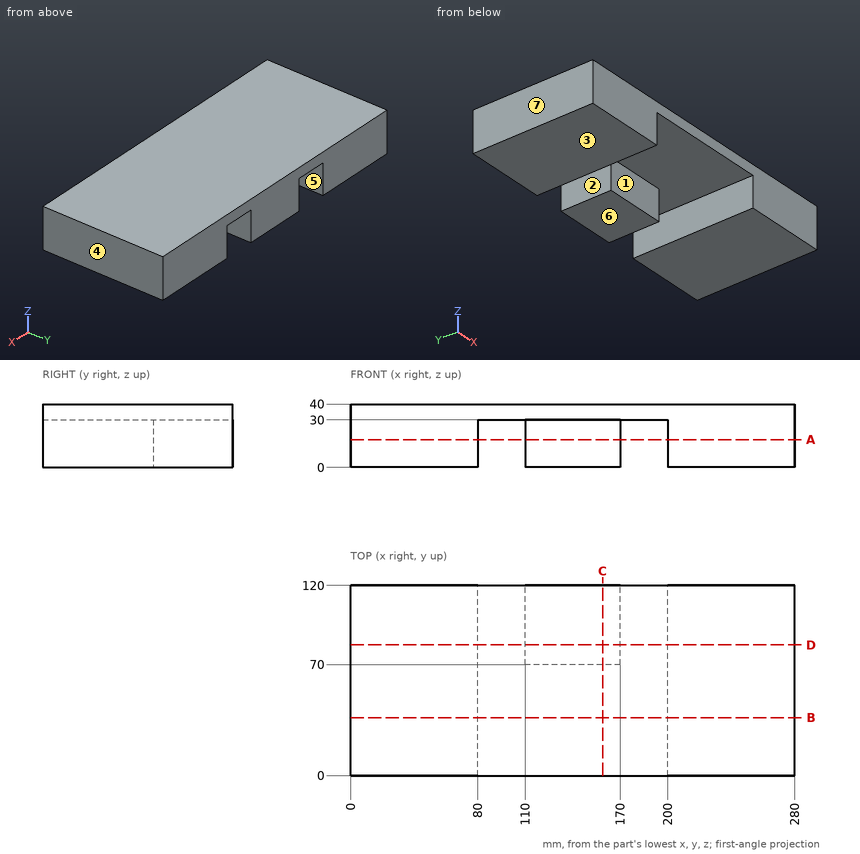
Geometry check sheet. Reference: drawing and pictorial views, mm from the part's lowest x, y, z. A direction names the side the tool comes from. Coordinates: 2 decimals unless noted, no trailing zeros. Loops run counter-clockwise (first coordinate to the right, second up) from the corner with the lowest first, then second, coordinate; pieces in that order, holes last. Notation, with made-up numbers: M 17.5,-12 L 33.5,-12 A14 cw 33.5,-8 Z; hole C 86,1.5 d10. An arc over 180 degrees is marked long. One line per item, written item: value.
1. Section check D-D on y = 82.5. Record the cut outline in (x, z).
Answers follow:
outline: M 0,0 L 80,0 L 80,30 L 110,30 L 110,0 L 170,0 L 170,30 L 200,30 L 200,0 L 280,0 L 280,40 L 0,40 Z
2. Section check A-A on z = 17.5. Record the cut outline in (x, y).
Answers follow:
outline: M 0,0 L 80,0 L 80,120 L 0,120 Z; M 110,70 L 170,70 L 170,120 L 110,120 Z; M 200,0 L 280,0 L 280,120 L 200,120 Z
3. Mould release check, pull along X, two halves, no side actions. Record for the marked faces 4, 5, 6 and 7: pulls with the +X half, pulls with the -X half, needs draft (parallel to the pull), parting line crosses it, or undercut.
Answers follow:
face 4: pulls with the +X half
face 5: undercut
face 6: needs draft
face 7: pulls with the -X half
4. Section check B-B on y = 36.5. Record the cut outline in (x, z).
Answers follow:
outline: M 0,0 L 80,0 L 80,30 L 200,30 L 200,0 L 280,0 L 280,40 L 0,40 Z
5. Gauge pin test, flat end, axial feed: P1, Ø24, axis at x = 130.5, z = 16.5, coming from the -Y side. Record the tip position at first contact, or that the pin passes through.
Answers follow:
P1: y = 70
6. Section check C-C on x = 159. Record the cut outline in (y, z), plus the area to 3 significant figures.
Answers follow:
outline: M 0,30 L 70,30 L 70,0 L 120,0 L 120,40 L 0,40 Z
area: 2,700 mm^2
7. Material ranges on line 1 along X through (y, z) = (74, 12); line 2 along X through (y, z) = (17, 9.5); line 3 along Y through (x, z) = (132, 18.5), recorded low to high. Write a range as from..to.
Answers follow:
line 1: 0..80, 110..170, 200..280
line 2: 0..80, 200..280
line 3: 70..120
8. Set-up check for the marked faces 1, 2 and 3: record each of +Z, -Z, +X, -X, +Y, -Y from which the full face is reachable in a straight line by a thin tool's end or side.
Answers follow:
face 1: -Z, -Y
face 2: -Z, +Y, -Y
face 3: -Z, +X, -X, +Y, -Y
